from build123d import *

# Parameters (mm, degrees)
F0_W     = 127
F0_H     = 127
F1_DEPTH = 127
F2_W     = 78.8183361292
F2_H     = 67.629866302
F3_DEPTH = 25.4
F4_T     = -2.54


with BuildPart() as f1:
    # F0 (on Front) → F1 (new body)
    with BuildSketch(Plane.XZ):
        with Locations((3.8867425174, 17.1191294668)):
            Rectangle(F0_W, F0_H)
    extrude(amount=F1_DEPTH)

    # F2 (on face) → F3 (join)
    with BuildSketch(Plane.XZ.offset(127)):
        Rectangle(F2_W, F2_H)
    extrude(amount=F3_DEPTH)

    # F4
    f4_openings = [f1.faces().sort_by_distance(p)[0] for p in [
        (0, -152.4, 0),
    ]]
    offset(amount=F4_T, openings=f4_openings, kind=Kind.INTERSECTION)


solid = f1.part
Geometry check sheet. Reference: the model listing, model coordinates, mm. A direction names the side the tool comes from. Round coordinates to 2 decimals unless told otherwise and drop trailing zeros. Loops run counter-clockwise (first coordinate to the right, second up) from the corner with the lowest first, then second, coordinate; pieces in that order, holes last. Notation, with made-up numbers: (29.25, 35.5) - (84.25, 35.5) arc R31 ccw to (84.25, 60.5) - close; hole circle Ø8 at (66, -19). An arc over 180 degrees is marked (long way). One line per question, with ' | ' between items. Start each with the question number.
1. Cross-section at A-A on y = -39.5. Record the cut outline in (x, z).
2. Cross-section at C-C on z = -38. Record the cut outline in (x, y), then the cut area to 3 significant figures.
3. Depth check by flat-ended pin: pin 1 (8.5 mm diameter, centred on y = -132, z = 7, fed in from +X); pin 2 (14 mm diameter, centred on y = -142, z = -12, fed in from -X); pin 3 (12.5 mm diameter, centred on x = 17.5, y = -135.5, fed in from +Z). Enter the tip coordinate at first touch or a pass-through.
4. Tool access check on faces 5 (the face through (3, -2.54, 18)), 6 (the face through (-1, -138, -31.275)), 7 (the face through (-39.409, -140, 0)). Record the directions out of +Z, -Z, +X, -X, +Y, -Y that give a thin tool (end or side, any length) a straight path to the whole face; none if there is none.
5. Draft check along X on faces 1 (the face through (-59.613, -63, 16)), 2 (the face through (-1, -138, 31.275)), 3 (the face through (3, -124.46, 32)), 4 (the face through (-1, -140, 33.815)). Enter one of: released by +X, released by -X, zero draft, split by the parting line, or undercut.
6. Cross-section at B-B on x = -11.5. Record the cut outline in (y, z).
7. Scan lines: line 1 (Y direction, x = 55.5, z = 43.5); line 2 (X direction, y = -106.5, z = -9); line 3 (Z direction, x = -16.5, y = -142.5). Record each from-to range of solid material in increasing order. Write a range as [from, to].
8. Cross-section at D-D on z = -17. Record the cut outline in (x, y).
Taken from the geometry:
1) outline: (-59.61, -46.38) - (67.39, -46.38) - (67.39, 80.62) - (-59.61, 80.62) - close; hole (-57.07, -43.84) - (64.85, -43.84) - (64.85, 78.08) - (-57.07, 78.08) - close
2) outline: (-59.61, -127) - (67.39, -127) - (67.39, 0) - (-59.61, 0) - close; hole (-57.07, -124.46) - (64.85, -124.46) - (64.85, -2.54) - (-57.07, -2.54) - close | area: 1,260 mm²
3) pin 1: x = 39.41 | pin 2: x = -39.41 | pin 3: z = 33.81
4) face 5: none | face 6: -Y | face 7: +Z, -Z, -X, -Y
5) face 1: released by -X | face 2: undercut | face 3: undercut | face 4: zero draft
6) outline: (-152.4, -33.81) - (-127, -33.81) - (-127, -46.38) - (0, -46.38) - (0, 80.62) - (-127, 80.62) - (-127, 33.81) - (-152.4, 33.81) - (-152.4, 31.27) - (-124.46, 31.27) - (-124.46, 78.08) - (-2.54, 78.08) - (-2.54, -43.84) - (-124.46, -43.84) - (-124.46, -31.27) - (-152.4, -31.27) - close
7) line 1: [-127, -124.46], [-2.54, 0] | line 2: [-59.61, -57.07], [64.85, 67.39] | line 3: [-33.81, -31.27], [31.27, 33.81]
8) outline: (-59.61, -127) - (-39.41, -127) - (-39.41, -152.4) - (-36.87, -152.4) - (-36.87, -124.46) - (-57.07, -124.46) - (-57.07, -2.54) - (64.85, -2.54) - (64.85, -124.46) - (36.87, -124.46) - (36.87, -152.4) - (39.41, -152.4) - (39.41, -127) - (67.39, -127) - (67.39, 0) - (-59.61, 0) - close
